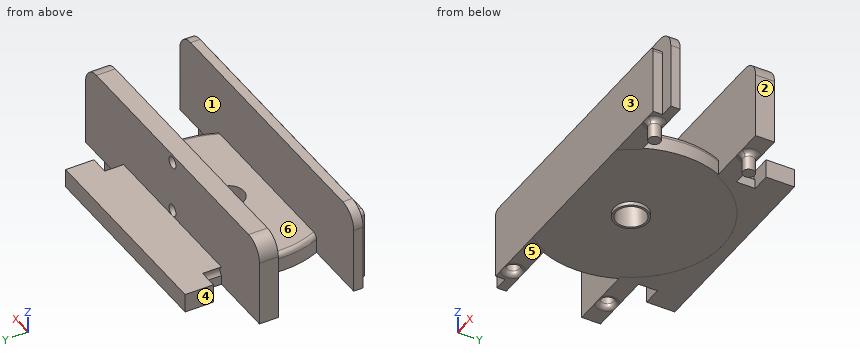
from build123d import *

# Parameters (mm, degrees)
BOSS_EXTRUDE1_DEPTH     = 2
SKETCH2_R               = 1.575
BOSS_EXTRUDE2_DEPTH     = 4
SKETCH3_R               = 1.8
BOSS_EXTRUDE3_DEPTH     = 0.4
SKETCH4_W               = 2
SKETCH4_H               = 17
BOSS_EXTRUDE4_DEPTH     = 0.001
SKETCH5_W               = 18
SKETCH5_H               = 2
BOSS_EXTRUDE5_DEPTH     = 0.001
SKETCH6_W               = 2.001
SKETCH6_H               = 2
BOSS_EXTRUDE6_DEPTH     = 5
BOSS_EXTRUDE7_DEPTH     = 0.001
CUT_EXTRUDE1_DEPTH      = 20.519323784
SKETCH9_W               = 2.937742252
SKETCH9_H               = 8
CUT_EXTRUDE2_DEPTH      = 0.001
CUT_EXTRUDE11_START     = -0.001
SKETCH21_R              = 9.75
SKETCH21_R_2            = 1.8
CUT_EXTRUDE11_DEPTH     = 0.001
SKETCH10_W              = 32
SKETCH10_H              = 2
BOSS_EXTRUDE8_DEPTH     = 7
FILLET1_R               = 0.5
SKETCH11_R              = 0.625
BOSS_EXTRUDE9_DEPTH     = 2
SKETCH14_W              = 2
SKETCH14_H              = 2
CUT_EXTRUDE5_DEPTH      = 22.401355237
SKETCH12_R              = 0.675
CUT_EXTRUDE3_DEPTH      = 2.5
CUT_EXTRUDE6_DEPTH      = 2
FILLET2_R               = 0.5
FILLET3_R               = 0.5
FILLET4_R               = 2
CUT_EXTRUDE7_DEPTH      = 26.019992106
CUT_EXTRUDE7_DEPTH_BACK = 1
SKETCH19_R              = 0.625
CUT_EXTRUDE9_DEPTH      = 2


with BuildPart() as part:
    # Sketch1 → Boss-Extrude1 (new body)
    with BuildSketch(Plane.XY):
        Polygon((-11, 6), (-11, 11), (11, 11), (11, 6), (11, -6), (-11, -6), align=None)
    extrude(amount=BOSS_EXTRUDE1_DEPTH)

    # Sketch3 → Boss-Extrude3 (add)
    with BuildSketch(Plane(origin=(0, 0, 0), x_dir=(-1, 0, 0), z_dir=(0, 0, -1))):
        with Locations(Location((0, 0, 0), (0, 0, 180))):
            Circle(SKETCH3_R)
    extrude(amount=BOSS_EXTRUDE3_DEPTH)

    # Sketch4 → Boss-Extrude4 (add)
    with BuildSketch(Plane(origin=(0, 0, 0), x_dir=(-1, 0, 0), z_dir=(0, 0, -1))):
        with Locations((10, 2.5)):
            Rectangle(SKETCH4_W, SKETCH4_H)
        with Locations((-10, 2.5)):
            Rectangle(SKETCH4_W, SKETCH4_H)
    extrude(amount=BOSS_EXTRUDE4_DEPTH)

    # Sketch5 → Boss-Extrude5 (add)
    with BuildSketch(Plane(origin=(0, 0, 0), x_dir=(-1, 0, 0), z_dir=(0, 0, -1))):
        with Locations((0, 10)):
            Rectangle(SKETCH5_W, SKETCH5_H)
    extrude(amount=BOSS_EXTRUDE5_DEPTH)

    # Sketch6 → Boss-Extrude6 (add)
    with BuildSketch(Plane(origin=(11, 0, 0), x_dir=(0, 0, -1), z_dir=(1, 0, 0))):
        with Locations((-0.9995, -5)):
            Rectangle(SKETCH6_W, SKETCH6_H)
        with Locations((-0.9995, 5)):
            Rectangle(SKETCH6_W, SKETCH6_H)
    boss_extrude6 = extrude(amount=BOSS_EXTRUDE6_DEPTH)

    # Mirror1: Boss-Extrude6 across plane
    add(boss_extrude6.mirror(Plane(origin=(0, 0, 0), x_dir=(0, 0, 1), z_dir=(1, 0, 0))))

    # Sketch7 → Boss-Extrude7 (add)
    with BuildSketch(Plane(origin=(0, 0, -0.001), x_dir=(-1, 0, 0), z_dir=(0, 0, -1))):
        with BuildLine():
            ThreePointArc((-6.708203932, -6), (-8.407551231, -3.211398808), (-9, 0))
            Line((-9, 0), (-9, -6))
            Line((-9, -6), (-6.708203932, -6))
        make_face()
        with BuildLine():
            Line((-9, 9), (-9, 0))
            ThreePointArc((-9, 0), (-6.363961031, 6.363961031), (0, 9))
            Line((0, 9), (-9, 9))
        make_face()
    boss_extrude7 = extrude(amount=-BOSS_EXTRUDE7_DEPTH)

    # Sketch8 → Cut-Extrude1 (cut, through all)
    with BuildSketch(Plane(origin=(0, 0, -0.001), x_dir=(-1, 0, 0), z_dir=(0, 0, -1))):
        with BuildLine():
            Line((-11, 4), (-9.16515139, 4))
            ThreePointArc((-9.16515139, 4), (-10, 0), (-9.16515139, -4))
            Line((-9.16515139, -4), (-11, -4))
            Line((-11, -4), (-11, 4))
        make_face()
    cut_extrude1 = extrude(amount=-CUT_EXTRUDE1_DEPTH, mode=Mode.SUBTRACT)

    # Sketch9 → Cut-Extrude2 (cut)
    with BuildSketch(Plane(origin=(0, 0, -0.001), x_dir=(-1, 0, 0), z_dir=(0, 0, -1))):
        with Locations((-9.531128874, 0)):
            Rectangle(SKETCH9_W, SKETCH9_H)
    cut_extrude2 = extrude(amount=-CUT_EXTRUDE2_DEPTH, mode=Mode.SUBTRACT)

    # Mirror2: Boss-Extrude7, Cut-Extrude1, Cut-Extrude2 across plane
    add(boss_extrude7.mirror(Plane(origin=(0, 0, 0), x_dir=(0, 0, 1), z_dir=(1, 0, 0))))
    add(cut_extrude1.mirror(Plane(origin=(0, 0, 0), x_dir=(0, 0, 1), z_dir=(1, 0, 0))), mode=Mode.SUBTRACT)
    add(cut_extrude2.mirror(Plane(origin=(0, 0, 0), x_dir=(0, 0, 1), z_dir=(1, 0, 0))), mode=Mode.SUBTRACT)

    # Sketch21 → Cut-Extrude11 (cut)
    with BuildSketch(Plane(origin=(0, 0, -0.001), x_dir=(-1, 0, 0), z_dir=(0, 0, -1)).offset(CUT_EXTRUDE11_START)):
        Circle(SKETCH21_R)
        with Locations(Location((0, 0, 0), (0, 0, 180))):
            Circle(SKETCH21_R_2, mode=Mode.SUBTRACT)
    extrude(amount=CUT_EXTRUDE11_DEPTH, mode=Mode.SUBTRACT)

    # Sketch10 → Boss-Extrude8 (add)
    with BuildSketch(Plane.XY.offset(2)):
        with Locations((0, -5)):
            Rectangle(SKETCH10_W, SKETCH10_H)
        with Locations((0, 5)):
            Rectangle(SKETCH10_W, SKETCH10_H)
    extrude(amount=BOSS_EXTRUDE8_DEPTH)

    # Fillet1
    fillet1_edges = [part.edges().sort_by_distance(p)[0] for p in [
        (10, 0, 2),
        (-10, 0, 2),
    ]]
    fillet(fillet1_edges, radius=FILLET1_R)

    # Sketch11 → Boss-Extrude9 (add)
    with BuildSketch(Plane(origin=(0, 0, -0.001), x_dir=(-1, 0, 0), z_dir=(0, 0, -1))):
        with Locations(Location((-13, -5, 0), (0, 0, 180))):
            Circle(SKETCH11_R)
    boss_extrude9 = extrude(amount=BOSS_EXTRUDE9_DEPTH)

    # Sketch14 → Cut-Extrude5 (cut, through all)
    with BuildSketch(Plane(origin=(0, 0, -0.001), x_dir=(-1, 0, 0), z_dir=(0, 0, -1))):
        with Locations((10, 7)):
            Rectangle(SKETCH14_W, SKETCH14_H)
        with Locations((-10, 7)):
            Rectangle(SKETCH14_W, SKETCH14_H)
    extrude(amount=-CUT_EXTRUDE5_DEPTH, mode=Mode.SUBTRACT)

    # Sketch12 → Cut-Extrude3 (cut)
    with BuildSketch(Plane(origin=(0, 0, -0.001), x_dir=(-1, 0, 0), z_dir=(0, 0, -1))):
        with Locations((13, -5)):
            Circle(SKETCH12_R)
    cut_extrude3 = extrude(amount=-CUT_EXTRUDE3_DEPTH, mode=Mode.SUBTRACT)

    # Sketch16 → Cut-Extrude6 (cut)
    with BuildSketch(Plane(origin=(0, 6, 0), x_dir=(1, 0, 0), z_dir=(0, 1, 0))):
        with BuildLine():
            Line((-9, -1), (-9, -2))
            ThreePointArc((-9, -2), (-8.75, -1.5), (-9, -1))
        make_face()
    cut_extrude6 = extrude(amount=CUT_EXTRUDE6_DEPTH, mode=Mode.SUBTRACT)

    # Mirror3: Boss-Extrude9, Cut-Extrude3 across plane
    add(boss_extrude9.mirror(Plane.ZX))
    add(cut_extrude3.mirror(Plane.ZX), mode=Mode.SUBTRACT)

    # Mirror4: Cut-Extrude6 across plane
    add(cut_extrude6.mirror(Plane(origin=(0, 0, 0), x_dir=(0, 0, 1), z_dir=(1, 0, 0))), mode=Mode.SUBTRACT)

    # Fillet2
    fillet2_edges = [part.edges().sort_by_distance(p)[0] for p in [
        (12.375, -5, -0.001),
        (12.375, 5, -0.001),
    ]]
    fillet(fillet2_edges, radius=FILLET2_R)

    # Fillet3
    # the kernel refuses this fillet: 0.5 mm, written as the material it takes off along each edge
    with BuildSketch(Plane(origin=(-13, -5, -0.001), x_dir=(-1, 0, 0), z_dir=(0, -1, 0))) as fillet3_piece_1:
        with BuildLine():
            CenterArc((0.675 + FILLET3_R, -FILLET3_R), FILLET3_R, 90, 90)
            Line((0.675, -FILLET3_R), (0.675, 0))
            Line((0.675, 0), (0.675 + FILLET3_R, 0))
        make_face()
    revolve(axis=Axis((-13, -5, -0.001), (0, 0, -1)), mode=Mode.SUBTRACT)
    with BuildSketch(Plane(origin=(-13, 5, -0.001), x_dir=(-1, 0, 0), z_dir=(0, 1, 0))) as fillet3_piece_2:
        with BuildLine():
            CenterArc((0.675 + FILLET3_R, FILLET3_R), FILLET3_R, 180, 90)
            Line((0.675, FILLET3_R), (0.675, 0))
            Line((0.675, 0), (0.675 + FILLET3_R, 0))
        make_face()
    revolve(axis=Axis((-13, 5, -0.001), (0, 0, 1)), mode=Mode.SUBTRACT)

    # Fillet4
    fillet4_edges = [part.edges().sort_by_distance(p)[0] for p in [
        (16, -5, 9),
        (-16, -5, 9),
        (-16, 5, 9),
        (16, 5, 9),
    ]]
    fillet(fillet4_edges, radius=FILLET4_R)

    # Sketch17 → Cut-Extrude7 (cut, two sides: drawn at the far end of the back side and taken through both)
    with BuildSketch(Plane.XZ.offset(6).offset(-CUT_EXTRUDE7_DEPTH_BACK)):
        with BuildLine():
            Line((-16, 7), (-16, -0.001))
            Line((-16, -0.001), (-14.5, -0.001))
            Line((-14.5, -0.001), (-14.5, 7))
            ThreePointArc((-14.5, 7), (-14.353553391, 7.353553391), (-14, 7.5))
            Line((-14, 7.5), (14, 7.5))
            ThreePointArc((14, 7.5), (14.353553391, 7.353553391), (14.5, 7))
            Line((14.5, 7), (14.5, -0.001))
            Line((14.5, -0.001), (16, -0.001))
            Line((16, -0.001), (16, 7))
            ThreePointArc((16, 7), (15.414213562, 8.414213562), (14, 9))
            Line((14, 9), (-14, 9))
            ThreePointArc((-14, 9), (-15.414213562, 8.414213562), (-16, 7))
        make_face()
    extrude(amount=CUT_EXTRUDE7_DEPTH + CUT_EXTRUDE7_DEPTH_BACK, mode=Mode.SUBTRACT)

    # Sketch19 → Cut-Extrude9 (cut)
    with BuildSketch(Plane(origin=(0, 6, 0), x_dir=(1, 0, 0), z_dir=(0, 1, 0))):
        with Locations(Location((0, -2.625, 0), (0, 0, 90))):
            Circle(SKETCH19_R)
        with Locations(Location((0, -8.125, 0), (0, 0, 270))):
            Circle(SKETCH19_R)
    extrude(amount=-CUT_EXTRUDE9_DEPTH, mode=Mode.SUBTRACT)


with BuildPart() as body_2:
    # Sketch2 → Boss-Extrude2 (new body)
    with BuildSketch(Plane(origin=(0, 0, 2), x_dir=(-1, 0, 0), z_dir=(0, 0, -1))):
        Circle(SKETCH2_R)
    extrude(amount=BOSS_EXTRUDE2_DEPTH)


with BuildPart() as part_1:
    add(part.part)

    # Combine2: cut body 2
    add(body_2.part, mode=Mode.SUBTRACT)


solid = part_1.part
Input: part model. Units: mm. Frame: model coordinates. Face numbers are marked on the shaded views. A direction names the side the tool comes from. Coordinates: 2 decimals unless noted, no trailing zeros. Loops run counter-clockwise (first coordinate to the right, second up) from the corner with the lowest first, then second, coordinate; pieces in that order, holes last.
(1) Section B-B on y = 5. Count the separate pieces of the cut face and the enclosed holes in it, then the cut area to 3 significant figures.
(2) First-contact query: pin 1 Ø1.6 at (x, y) = (-10, -5.5) entering from -Z; pin 2 Ø6 at (x, z) = (6.5, 5.5) entering from +Y; pin 3 Ø2.5 at (x, y) = (0, 0) entering from -Z. Flat tips, straight axial feed; report the tip coordinate or a pass-through.
(3) Pull-direction query (Y, two-part tool) for the marked faces 1, 2 and 3; classes: released by +Y, released by -Y, zero draft, split by the parting line, or undercut.
(4) Section A-A on x = -13. Return the cut outline in (y, z) (3 decimals).
(5) Material intervals for probe 1 along Y at (x, z) = (-13, 1) (3 decimals); probe 2 along Y at (x, z) = (6.5, 4.25); probe 3 along Y at (x, z) = (-1.5, 7.75), sorted ascending.
(6) Set-up query: the marked faces 4, 5 and 6. Return all of +Z, -Z, +X, -X, +Y, -Y with unobstructed straight access to the full face (end or side cutting, diameter ignored); none if empty.
Data:
1. separate pieces: 1
1. enclosed holes: 2
1. area: 283 mm2
2. pin 1: stops at z = 0
2. pin 2: stops at y = 6
2. pin 3: passes through
3. face 1: undercut
3. face 2: zero draft
3. face 3: released by -Y
4. outline: (-6, 0.031) arc R0.5 ccw to (-5.675, 0.499) - (-5.675, 2.499) - (-4.325, 2.499) - (-4.325, 0.499) arc R0.5 ccw to (-4, 0.031) - (-4, 9) - (-5, 9) - (-5, 7.5) - (-6, 7.5) - close; (4, 0.031) arc R0.5 ccw to (4.325, 0.499) - (4.325, 2.499) - (5.675, 2.499) - (5.675, 0.499) arc R0.5 ccw to (6, 0.031) - (6, 9) - (4, 9) - close
5. probe 1: y = -6 to -5.675, -4.325 to -4, 4 to 4.325, 5.675 to 6
5. probe 2: y = -6 to -4, 4 to 6
5. probe 3: y = -5 to -4, 4 to 6
6. face 4: +Z, -Z, -X, +Y
6. face 5: -Z, -X, +Y, -Y
6. face 6: +Z, +X, -X
